Design review of the part built by this model. Coordinates are the model's own, in mm. A direction names the side the tool comes from. Give positions to 0.01 mm unless a question says otherwise; leave off trailing zeros. Loops run counter-clockwise (first coordinate to the right, second up) from the corner with the lowest first, then second, coordinate; pieces in that order, holes last.
from build123d import *

# Parameters (mm, degrees)
SKETCH1_W            = 1.5875
SKETCH1_H            = 22.225
M4_CLEARANCE_HOLE1_D = 4.8


with BuildPart() as part:
    # Sketch1 → Revolve1 (revolve)
    with BuildSketch(Plane.XY):
        Polygon((0, 25.4), (0, 22.225), (1.5875, 22.225), (12.7, 22.225), (12.7, 25.4), align=None)
        Polygon((-1.5875, 22.225), (0, 22.225), (0, 25.4), (-12.7, 25.4), (-12.7, 22.225), align=None)
        with Locations((-0.79375, 11.1125)):
            Rectangle(SKETCH1_W, SKETCH1_H)
        with Locations((0.79375, 11.1125)):
            Rectangle(SKETCH1_W, SKETCH1_H)
    revolve(axis=Axis((0, 0, 0), (1, 0, 0)))

    # M4 Clearance Hole1 (through all)
    with Locations(Plane.ZY.offset(1.5875)):
        with Locations((0, 0)):
            Hole(M4_CLEARANCE_HOLE1_D / 2)


solid = part.part
Q1. Take a section at C-C (x = 3.75). Give the boundary of the cut face in (y, z) (3 decimals), plus the area to 3 significant figures.
Results:
outline: circle Ø50.8 at (0, 0); hole circle Ø44.45 at (0, 0)
area: 475 mm2
Q2. Take a section at D-D (y = -14). Give the boundary of the cut face in (x, z).
Results:
outline: (-12.7, -21.19) - (12.7, -21.19) - (12.7, -17.26) - (1.59, -17.26) - (1.59, 17.26) - (12.7, 17.26) - (12.7, 21.19) - (-12.7, 21.19) - (-12.7, 17.26) - (-1.59, 17.26) - (-1.59, -17.26) - (-12.7, -17.26) - close
Q3. Wall thickness on line 1 (Z direction, x = 10.75, y = 0) (3 decimals); line 2 (X direction, y = -3.5, z = -10); line 3 (Y direction, x = 11.5, z = -16): over which ranges is each line inside the solid? List them lowest first.
Results:
line 1: z = -25.4 to -22.225, 22.225 to 25.4
line 2: x = -1.59 to 1.59
line 3: y = -19.73 to -15.43, 15.43 to 19.73
Q4. Tool access review of faces 1 (the face through (7.222, 21.199, 6.676)), 2 (the face through (-1.588, 0, -5)), 3 (the face through (0.022, 2.024, -1.29)): name each direction out of +Z, -Z, +X, -X, +Y, -Y from which nothing blocks a thin tool from reaching the whole face with its end or side.
Results:
face 1: +X
face 2: -X
face 3: +X, -X
Q5. Draft analysis for pull direction Y (two halves, no side actions). For faces 4 (the face through (-0.178, -5.506, -24.796)), 5 (the face through (12.7, 0.1, -22.5)), 6 (the face through (-7.066, 21.199, 6.676)), state which applies: pulls with the +Y half, pulls with the -Y half, needs draft (parallel to the pull), parting line crosses it, or undercut.
Results:
face 4: parting line crosses it
face 5: needs draft
face 6: undercut
Q6. Insertion check: pin 1 (4 mm diameter, centred on x = 5.5, z = -11, fed in from +Y); pin 2 (6 mm diameter, centred on y = -10, z = 9, fed in from -X); pin 3 (6 mm diameter, centred on y = 0, z = 0, fed in from +X). Each pin has a flat end and moves straight along its axis. Give the tip position at first contact, or say it passes through.
Results:
pin 1: stops at y = 23.75
pin 2: stops at x = -1.59
pin 3: stops at x = 1.59
Q7. Take a section at A-A (y = 0). Give the boundary of the cut face in (x, z) (1 decimal).
Results:
outline: (-12.7, -25.4) - (12.7, -25.4) - (12.7, -22.2) - (1.6, -22.2) - (1.6, -2.4) - (-1.6, -2.4) - (-1.6, -22.2) - (-12.7, -22.2) - close; (-12.7, 22.2) - (-1.6, 22.2) - (-1.6, 2.4) - (1.6, 2.4) - (1.6, 22.2) - (12.7, 22.2) - (12.7, 25.4) - (-12.7, 25.4) - close
